```python
from build123d import *

# Parameters (mm, degrees)
F0_W     = 8
F0_H     = 30
F2_DEPTH = 9.25
F4_DEPTH = 32.5
F5_W     = 17.5
F5_H     = 15
F6_DEPTH = 30


with BuildPart() as f1:
    # F0 (on Front) → F1 (revolve)
    with BuildSketch(Plane.XZ):
        Polygon((21.4039260229, 59.6839201814), (25.9981002354, 34.6839201814), (24.4039260229, 59.6839201814), align=None)
        Polygon((24.4039260229, 59.6839201814), (25.9981002354, 67.1839201814), (22.9981002354, 67.1839201814), (21.4039260229, 59.6839201814), align=None)
        Polygon((22.9981002354, 67.1839201814), (25.9981002354, 67.1839201814), (24.83233109, 69.6839201814), (22.9981002354, 69.6839201814), align=None)
        Polygon((21.83233109, 69.6839201814), (22.9981002354, 67.1839201814), (22.9981002354, 69.6839201814), align=None)
        Polygon((24.4039260229, 59.6839201814), (25.9981002354, 34.6839201814), (25.9981002354, 67.1839201814), align=None)
    revolve(axis=Axis((17.9981002354, 0, 37.1839201814), (0, 0, 1)))

    # F0 (on Front) → F2 (join, symmetric)
    with BuildSketch(Plane.XZ):
        Polygon((7.4981002354, 4.6839201814), (9.9981002354, 4.6839201814), (9.9981002354, 34.6839201814), (9.9981002354, 67.1839201814), (7.4981002354, 67.1839201814), align=None)
        Polygon((25.9981002354, 34.6839201814), (25.9981002354, 4.6839201814), (28.4981002354, 4.6839201814), (28.4981002354, 67.1839201814), (25.9981002354, 67.1839201814), align=None)
        with Locations((13.9981002354, 19.6839201814)):
            Rectangle(F0_W, F0_H)
        with Locations((21.9981002354, 19.6839201814)):
            Rectangle(F0_W, F0_H)
    extrude(amount=F2_DEPTH, both=True)

    # F3 (on face) → F4 (join, through all)
    with BuildSketch(Plane.XY.offset(34.6839201814)):
        with BuildLine():
            Line((25.9981002354, -9.25), (25.9981002354, 0))
            ThreePointArc((25.9981002354, 0), (17.998100241, -8), (9.9981002354, -1.11e-08))
            Line((9.9981002354, -1.11e-08), (9.9981002354, -9.25))
            Line((9.9981002354, -9.25), (25.9981002354, -9.25))
        make_face()
        with BuildLine():
            ThreePointArc((9.9981002354, -1.11e-08), (17.9981002299, 8), (25.9981002354, 0))
            Line((25.9981002354, 0), (25.9981002354, 9.25))
            Line((25.9981002354, 9.25), (9.9981002354, 9.25))
            Line((9.9981002354, 9.25), (9.9981002354, -1.11e-08))
        make_face()
    extrude(amount=F4_DEPTH)

    # F5 (on face) → F6 (cut)
    with BuildSketch(Plane(origin=(0, 0, 4.6839201814), x_dir=(1, 0, 0), z_dir=(0, 0, -1))):
        with Locations((17.9981002354, 0)):
            Rectangle(F5_W, F5_H)
    extrude(amount=-F6_DEPTH, mode=Mode.SUBTRACT)


solid = f1.part
```
Can you work these out from the model? Positions are in its coordinate system, mm. A direction names the side the tool comes from. Give positions to 0.01 mm unless a question says otherwise; leave off trailing zeros. Order: outer loops, then holes, each group sorted by start corner. A loop starts at its lowest first (then second) coordinate and runs counter-clockwise, first axis right, second up. Notation, with made-up numbers: (19.5, 75) - (45.5, 75) arc R25 cw to (45.5, 103) - close; hole circle Ø3 at (62.25, 65). An arc over 180 degrees is marked (long way). Use a Markdown table: item, result. Add a question column.
Q1. I'm going to push a flat-ended pin straight in: pin 1 (1.8 mm diameter, centred on x = 11, y = 3, fed in from -Z). Where does the tip first touch, or does it pass through?
Q2. If we section it at B-B on y = 0: Write out the boundary of the cut face in (x, z).
Q3. Please list where these lines run through material, in increasing order: line 1 along X through (y, z) = (-6.5, 20); line 2 along Y through (x, z) = (12, 16.5); line 3 along Z through (x, y) = (8.75, 5).
Q4. On a 3-axis mill with a long thin cutter (end or side, diameter ignored), from which of +Z, -Z, +X, -X, +Y, -Y can I reach the whole of each face in a straight line? I mean faces 1 (the flat face through (18, -7.5, 19)), 2 (the flat face through (10.9, 4.2, 67.184)), 3 (the flat face through (7.498, 0, 36)), 4 (the conical face through (14, 0.2, 62.5)). Say none if no direction works.
Q5. If we section it at C-C on z = 36.5: Write out the boundary of the cut face in (x, y).
Q6. If we mould it in two halves opening along X, with no side actions, what happens to faces 5 (the flat face through (26.2, 0.5, 34.684)), 6 (the flat face through (28.498, 0, 35)), 7 (the flat face through (18, 9.25, 36)), 8 (the flat face through (9.248, 0, 19))? For each: released by +X, released by -X, zero draft, split by the parting line, or undercut.
Q7. If we section it at A-A on z = 16.5: Write out the boundary of the cut face in (x, y), plus the area to 3 significant figures.
Answers follow:
| question | item | result |
|---|---|---|
| 1 | pin 1 | stops at z = 34.68 |
| 2 | outline | (7.5, 4.68) - (9.25, 4.68) - (9.25, 34.68) - (10, 34.68) - (14.59, 59.68) - (13, 67.18) - (14.16, 69.68) - (11.16, 69.68) - (10, 67.18) - (7.5, 67.18) - close; (21.4, 59.68) - (26, 34.68) - (26.75, 34.68) - (26.75, 4.68) - (28.5, 4.68) - (28.5, 67.18) - (26, 67.18) - (24.83, 69.68) - (21.83, 69.68) - (23, 67.18) - close |
| 3 | line 1 | x = 7.5 to 9.25, 26.75 to 28.5 |
| 3 | line 2 | y = -9.25 to -7.5, 7.5 to 9.25 |
| 3 | line 3 | z = 4.68 to 67.18 |
| 4 | face 1 | -Z |
| 4 | face 2 | +Z |
| 4 | face 3 | +Z, -Z, -X, +Y, -Y |
| 4 | face 4 | none |
| 5 | outline | (7.5, -9.25) - (28.5, -9.25) - (28.5, 9.25) - (7.5, 9.25) - close; hole circle Ø15.33 at (18, 0) |
| 6 | face 5 | undercut |
| 6 | face 6 | released by +X |
| 6 | face 7 | zero draft |
| 6 | face 8 | undercut |
| 7 | outline | (7.5, -9.25) - (28.5, -9.25) - (28.5, 9.25) - (7.5, 9.25) - close; hole (9.25, -7.5) - (26.75, -7.5) - (26.75, 7.5) - (9.25, 7.5) - close |
| 7 | area | 126 mm^2 |
